```python
from build123d import *

# Parameters (mm, degrees)
SKETCH1_R           = 1.6
SKETCH1_R_2         = 12.25
BOSS_EXTRUDE1_DEPTH = 2.5


with BuildPart() as part:
    # Sketch1 → Boss-Extrude1 (new body)
    with BuildSketch(Plane.XY.offset(1.25)):
        with BuildLine():
            Line((-21, 18), (-21, -18))
            ThreePointArc((-21, -18), (-20.414213562, -19.414213562), (-19, -20))
            Line((-19, -20), (19, -20))
            ThreePointArc((19, -20), (20.414213562, -19.414213562), (21, -18))
            Line((21, -18), (21, 18))
            ThreePointArc((21, 18), (20.414213562, 19.414213562), (19, 20))
            Line((19, 20), (-19, 20))
            ThreePointArc((-19, 20), (-20.414213562, 19.414213562), (-21, 18))
        make_face()
        with Locations(Location((-15.5, 15.5, 0), (0, 0, 180))):
            Circle(SKETCH1_R, mode=Mode.SUBTRACT)
        with Locations(Location((15.5, -15.5, 0), (0, 0, 180))):
            Circle(SKETCH1_R, mode=Mode.SUBTRACT)
        with Locations(Location((0, 0, 0), (0, 0, 180))):
            Circle(SKETCH1_R_2, mode=Mode.SUBTRACT)
        with Locations(Location((-15.5, -15.5, 0), (0, 0, 180))):
            Circle(SKETCH1_R, mode=Mode.SUBTRACT)
        with Locations(Location((15.5, 15.5, 0), (0, 0, 180))):
            Circle(SKETCH1_R, mode=Mode.SUBTRACT)
    extrude(amount=-BOSS_EXTRUDE1_DEPTH)


solid = part.part
```
The listing builds one solid part. Answer for the finished solid, in the listing's coordinates (mm). Coordinates: 2 decimals unless noted, no trailing zeros. Write each loop counter-clockwise with the first axis right and the second up, starting at its lowest first coordinate (ties: lowest second). Pieces come first, ordered by that corner, then holes.
Q1. The mould has two halves that part along X. Classify faces 1 (the flat face through (-21, 0, 0)), 2 (the flat face through (21, 0, 0)), 3 (the cylindrical face through (-14.32, -16.58, 0.02)), 4 (the cylindrical face through (-6.586, -10.329, 0.018)): released by +X, released by -X, zero draft, split by the parting line, or undercut.
Returned:
face 1: released by -X
face 2: released by +X
face 3: undercut
face 4: undercut
Q2. Section D-D, the plane z = -0.3 is taken. Write down the section's boundary in (x, y), then the cut area to 3 significant figures.
Returned:
outline: (-21, -18) arc R2 ccw to (-19, -20) - (19, -20) arc R2 ccw to (21, -18) - (21, 18) arc R2 ccw to (19, 20) - (-19, 20) arc R2 ccw to (-21, 18) - close; hole circle Ø3.2 at (-15.5, -15.5); hole circle Ø3.2 at (-15.5, 15.5); hole circle Ø24.5 at (0, 0); hole circle Ø3.2 at (15.5, -15.5); hole circle Ø3.2 at (15.5, 15.5)
area: 1,170 mm2
Q3. Section C-C, the plane y = 15.5 is taken. Write down the section's boundary in (x, z), then the cut area to 3 significant figures.
Returned:
outline: (-21, -1.25) - (-17.1, -1.25) - (-17.1, 1.25) - (-21, 1.25) - close; (-13.9, -1.25) - (13.9, -1.25) - (13.9, 1.25) - (-13.9, 1.25) - close; (17.1, -1.25) - (21, -1.25) - (21, 1.25) - (17.1, 1.25) - close
area: 89.0 mm2
Q4. Section A-A, the plane x = 0 is taken. Write down the section's boundary in (y, z), then the cut area to 4 significant figures.
Returned:
outline: (-20, -1.25) - (-12.25, -1.25) - (-12.25, 1.25) - (-20, 1.25) - close; (12.25, -1.25) - (20, -1.25) - (20, 1.25) - (12.25, 1.25) - close
area: 38.75 mm2
Q5. Section B-B, the plane x = -15.5 is taken. Write down the section's boundary in (y, z), then the cut area to 3 significant figures.
Returned:
outline: (-20, -1.25) - (-17.1, -1.25) - (-17.1, 1.25) - (-20, 1.25) - close; (-13.9, -1.25) - (13.9, -1.25) - (13.9, 1.25) - (-13.9, 1.25) - close; (17.1, -1.25) - (20, -1.25) - (20, 1.25) - (17.1, 1.25) - close
area: 84.0 mm2
Q6. Given P1, Ø1.9, axis at x = 15.5, y = -15.5, coming from the +Z side; P2, Ø4, axis at x = 15.5, y = 15.5, coming from the +Z side, each flat-ended and moving along its own axis, determine where each tip first touches the part or whether it passes through.
Returned:
P1: passes through
P2: stops at z = 1.25
Q7. Find the intervals of material crossed by line 1 along X through (y, z) = (15.5, -0.45); line 2 along Y through (x, z) = (15.5, 0.7); line 3 along Y through (x, z) = (-0.5, 1.1), in increasing order.
Returned:
line 1: x = -21 to -17.1, -13.9 to 13.9, 17.1 to 21
line 2: y = -20 to -17.1, -13.9 to 13.9, 17.1 to 20
line 3: y = -20 to -12.24, 12.24 to 20
